CAD build for the part. Positions are in the model's coordinates, mm. A direction names the side the tool comes from. Round coordinates to 2 decimals unless told otherwise and drop trailing zeros. Loops run counter-clockwise (first coordinate to the right, second up) from the corner with the lowest first, then second, coordinate; pieces in that order, holes last. Notation, with made-up numbers: M 17.25,89 L 53.25,89 A19 ccw 53.25,96 Z; hole C 46,-19 d4. An arc over 180 degrees is marked long. Use a Markdown table: item, result. Add a question column.
(1) Flat gauge pins, fed straight in: P1, Ø4, axis at x = -66, y = -40, coming from the -Z side; P2, Ø2.5, axis at y = -111, z = 4, coming from the +X side; P3, Ø4, axis at x = 62.5, z = 6, coming from the +Y side; P4, Ø1.5, axis at x = -58.5, z = 4.5, coming from the +Y side. Where does each tip first touch, or does it go through?
(2) Two-plate mould, pull along Y, no slides. Class faces 1 (the face through (-86.5, 2, 4)), 2 (the face through (-3.5, -115, 4)), 3 (the face through (-71.3, 148.2, 3.9)), 4 (the face through (-71.7, -147.8, 3.9)): released by +Y, released by -Y, zero draft, split by the parting line, or undercut.
(3) Band-saw the part on A-A, the plane z = 4.5. Write the cut outline in (x, y), and give its area (3 significant figures).
(4) Which spindle directions (+Z, -Z, +X, -X, +Y, -Y) get a long thin tool onto all of the face, cutting with end or side? Do faces 5 (the face through (42, -125, 4)), 6 (the face through (38.91, 20.16, 3.94)), 7 (the face through (41, 155, 4)). Say none if no direction does.
(5) Band-saw the part on C-C, the plane x = 46.5. Write the cut outline in (y, z), and give its area (3 significant figures).
(6) Wall check: L1, parallel to Y at x = 46.5, z = 1.5; L2, parallel to X at y = 95, z = 3; L3, parallel to X at y = -52, z = 0.75. Give the ranges that are in metal, low to high.
(7) Band-saw the part on B-B, the plane y = -45. Write the cut outline in (x, z).
Autodesk Fusion 360 part; units mm, degrees
sketch "スケッチ1" plane through (0, 0, 0) normal (0, 0, 1) x (1, 0, 0)
  line L0 (-3.5, 163) -> (-86.5, 163)
  line L1 (-86.5, 163) -> (-86.5, -163)
  line L2 (-86.5, -163) -> (-3.5, -163)
  line L3 (86.5, -105) -> (86.5, 155)
  line L4 (82.2546, 155) -> (-86.5, -163) construction
  line L5 (-3.5, 163) -> (-3.5, 155)
  line L6 (-3.5, 155) -> (86.5, 155)
  line L7 (-86.5, -163) -> (-3.5, -163) construction
  line L8 (-3.5, -163) -> (86.5, -125)
  line L9 (86.5, -125) -> (-3.5, -125)
  line L10 (-3.5, -125) -> (-3.5, -105)
  line L11 (-3.5, -105) -> (86.5, -105)
  line L12 (-86.5, 163) -> (55.7209, -105) construction
  line L13 (66.3344, -125) -> (70.0256, -131.9558) construction
  dimension "d2" = 326
  dimension "d5" = 83
  dimension "d7" = 90
  dimension "d8" = 20
extrude "押し出し1" add sketch "スケッチ1" along normal blind 8
chamfer "面取り1" distance 30 angle 45 2 edges at (-86.5, -163, 4) (-86.5, 163, 4)
sketch "スケッチ2" plane through (0, 0, 8) normal (0, 0, 1) x (-1, 0, 0)
  line L0 (56.5, -163) -> (86.5, -133)
  line L1 (86.5, -133) -> (86.5, 133)
  line L2 (86.5, 133) -> (56.5, 163)
  line L3 (56.5, 163) -> (3.5, 163)
  line L4 (3.5, 163) -> (-86.5, 125)
  line L5 (-86.5, 125) -> (3.5, 125)
  line L6 (3.5, 125) -> (3.5, 105)
  line L7 (3.5, 105) -> (-86.5, 105)
  line L8 (-86.5, 105) -> (-86.5, -155)
  line L9 (-86.5, -155) -> (3.5, -155)
  line L10 (3.5, -155) -> (3.5, -163)
  line L11 (3.5, -163) -> (56.5, -163)
  line L12 (-86.5, -155) -> (-46.5, -155) construction
  line L13 (-46.5, -155) -> (-46.5, -95) construction
  line L14 (-46.5, -95) -> (-86.5, -95) construction
  line L15 (-86.5, -95) -> (-86.5, -155) construction
  line L16 (-46.5, -95) -> (-46.5, -25) construction
  line L17 (-46.5, -25) -> (-46.5, 45) construction
  point P0 (-46.5, -95)
  point P1 (-46.5, -25)
  point P2 (-46.5, 45)
  dimension "d12" = 40
  dimension "d13" = 60
  dimension "d14" = 70
  dimension "d15" = 70
hole "穴1" at (46.5, 95, 8) at (46.5, 25, 8) at (46.5, -45, 8) direction (0, 0, -1) diameter 18 end through all
equation "d5 = 30 mm + 53 mm"
Return value:
| question | item | result |
|---|---|---|
| 1 | P1 | z = 0 |
| 1 | P2 | x = -3.5 |
| 1 | P3 | y = 155 |
| 1 | P4 | y = 161.75 |
| 2 | face 1 | zero draft |
| 2 | face 2 | undercut |
| 2 | face 3 | released by +Y |
| 2 | face 4 | released by -Y |
| 3 | outline | M -86.5,-133 L -56.5,-163 L -3.5,-163 L 86.5,-125 L -3.5,-125 L -3.5,-105 L 86.5,-105 L 86.5,155 L -3.5,155 L -3.5,163 L -56.5,163 L -86.5,133 Z; hole C 46.5,-45 d18; hole C 46.5,25 d18; hole C 46.5,95 d18 |
| 3 | area | 50,500 mm^2 |
| 4 | face 5 | +Z, -Z, +X |
| 4 | face 6 | +Z, -Z |
| 4 | face 7 | +Z, -Z, +X, +Y |
| 5 | outline | M -141.89,0 L -125,0 L -125,8 L -141.89,8 Z; M -105,0 L -54,0 L -54,8 L -105,8 Z; M -36,0 L 16,0 L 16,8 L -36,8 Z; M 34,0 L 86,0 L 86,8 L 34,8 Z; M 104,0 L 155,0 L 155,8 L 104,8 Z |
| 5 | area | 1,780 mm^2 |
| 6 | L1 | -141.89 to -125, -105 to -54, -36 to 16, 34 to 86, 104 to 155 |
| 6 | L2 | -86.5 to 37.5, 55.5 to 86.5 |
| 6 | L3 | -86.5 to 40.84, 52.16 to 86.5 |
| 7 | outline | M -86.5,0 L 37.5,0 L 37.5,8 L -86.5,8 Z; M 55.5,0 L 86.5,0 L 86.5,8 L 55.5,8 Z |
